Design review of the part built by this model. Coordinates are the model's own, in mm. A direction names the side the tool comes from. Give positions to 0.01 mm unless a question says otherwise; leave off trailing zeros. Order: outer loops, then holes, each group sorted by start corner. A loop starts at its lowest first (then second) coordinate and runs counter-clockwise, first axis right, second up. Notation, with made-up numbers: (-7.5, 77) -> (28.5, 77) arc R28 cw to (28.5, 109) -> close; hole circle Ø10 at (30, -27.75). An arc over 180 degrees is marked (long way). One line per item, written item: value.
from build123d import *

# Parameters (mm, degrees)
F1_DEPTH = 25.4
F2_DEPTH = 6.35
F3_DEPTH = 6.35
F4_SIZE2 = 6.35
F4_SIZE  = 3.175
F5_SIZE2 = 3.175
F5_SIZE  = 6.35


with BuildPart() as f1:
    # F0 (on Top) → F1 (new body)
    with BuildSketch(Plane.XY):
        Polygon((25.4, 25.4), (25.4, -25.4), (-25.4, -25.4), (-31.75, -25.4), (-31.75, -31.75), (31.75, -31.75), (31.75, 31.75), (25.4, 31.75), align=None)
    extrude(amount=F1_DEPTH)

    # F2 (add): a face of the model
    f2_faces = [f1.faces().sort_by_distance(p)[0] for p in [
        (-31.75, -28.575, 12.7),
    ]]
    extrude(f2_faces, amount=F2_DEPTH)

    # F3 (add): a face of the model
    f3_faces = [f1.faces().sort_by_distance(p)[0] for p in [
        (28.575, 31.75, 12.7),
    ]]
    extrude(f3_faces, amount=F3_DEPTH)

    # F4
    f4_edges = [f1.edges().sort_by_distance(p)[0] for p in [
        (-38.1, -25.4, 12.7),
    ]]
    chamfer(f4_edges, length=F4_SIZE, length2=F4_SIZE2)

    # F5
    f5_edges = [f1.edges().sort_by_distance(p)[0] for p in [
        (25.4, 38.1, 12.7),
    ]]
    chamfer(f5_edges, length=F5_SIZE, length2=F5_SIZE2)


solid = f1.part
Item 1: Clearance check with flat-ended pins moving along their axes: P1, Ø8, axis at x = -27, z = 7, coming from the +Y side; P2, Ø1.5, axis at y = 2, z = 12.5, coming from the -X side. State where each tip first meets the part, or that it passes through.
Returned:
P1: y = -25.4
P2: x = 25.4
Item 2: Add section A-A on z = 2.25. Give the boundary of the cut face in (x, y) (3 decimals).
Returned:
outline: (-38.1, -31.75) -> (31.75, -31.75) -> (31.75, 38.1) -> (28.575, 38.1) -> (25.4, 31.75) -> (25.4, -25.4) -> (-31.75, -25.4) -> (-38.1, -28.575) -> close
Item 3: To check wall thickness, follow line 1 along Y through (x, z) = (-4.5, 13.25); line 2 along X through (y, z) = (11, 3.5). State the ranges of each line that lie inside material, in increasing order. Write a range as from..to.
Returned:
line 1: -31.75..-25.4
line 2: 25.4..31.75
Item 4: Add section C-C on y = -23.5. Give the boundary of the cut face in (x, z), plus the area to 3 significant figures.
Returned:
outline: (25.4, 0) -> (31.75, 0) -> (31.75, 25.4) -> (25.4, 25.4) -> close
area: 161 mm²
Item 5: Add section B-B on x = -30.5. Give the boundary of the cut face in (y, z).
Returned:
outline: (-31.75, 0) -> (-25.4, 0) -> (-25.4, 25.4) -> (-31.75, 25.4) -> close
Item 6: Machinability: for faces 1 (the flat face through (30, 38.1, 13)), 2 (the flat face through (25.4, 3, 13)), which of the approach directions +Z, -Z, +X, -X, +Y, -Y give a long, thin tool a straight path to every point of the face, cutting with its end or side? Answer none if there is none.
Returned:
face 1: +Z, -Z, +X, -X, +Y
face 2: +Z, -Z, -X, +Y
